Here's how the part is built. I have some questions about the finished solid (model axes, mm). A direction names the side the tool comes from. Coordinates: 2 decimals unless noted, no trailing zeros. Write each loop counter-clockwise with the first axis right and the second up, starting at its lowest first coordinate (ties: lowest second). Pieces come first, ordered by that corner, then holes. Notation, with made-up numbers: (66.25, 69.25) -> (94.25, 69.25) arc R20 cw to (94.25, 90.25) -> close; hole circle Ø9 at (-25.5, 34). An arc over 180 degrees is marked (long way). Use a Markdown table: item, result. Add a question column.
Item 1: Imagine slicing it at A-A, the plane x = 0. Write out the boundary of the cut face in (y, z).
Item 2: Will these pins go through, and if not, where does the flat tip stop? pin 1 Ø4 at (x, z) = (-36, -63) entering from +Y; pin 2 Ø2 at (x, z) = (-5, 24.3) entering from +Y; pin 3 Ø8 at (y, z) = (9, 56) entering from +X; pin 4 Ø6 at (x, z) = (-74.65, 0) entering from +Y.
Item 3: If I drill on line 1 along X through (y, z) = (3, 0); line 2 along X through (y, z) = (26, 34); line 3 along Z through (x, y) = (5, 25.5), over which ranges is the centre line in solid material (lowest first)? Write a range as from..to.
Item 4: Imagine slicing it at C-C, the plane z = 47.5. Write out the boundary of the cut face in (x, y).
Item 5: On a 3-axis mill with a long thin cutter (end or side, diameter ignored), from which of +Z, -Z, +X, -X, +Y, -Y can I reach the whole of each face in a straight line? I mean faces 1 (the flat face through (0, 20, 20.574)), 2 (the flat face through (-10.16, 5, -1)), 3 (the flat face through (43, 53.34, -29)). Say none if no direction works.
Item 6: Imagine slicing it at B-B, the plane z = 0. Write out the boundary of the cut face in (x, y).
Item 7: Imagine slicing it at D-D, the plane y = 35. Write out the boundary of the cut face in (x, z).
Item 8: If we mould it in two halves opening along Z, with no side actions, what happens to faces 4 (the flat face through (61.13, 6.858, 17.84)), 5 (the flat face through (0, 7.366, 0)), 6 (the cylindrical face through (81.318, 3.381, -10.677))? For each: pulls with the +Z half, pulls with the -Z half, needs draft (parallel to the pull), parting line crosses it, or undercut.
```python
from build123d import *

# Parameters (mm, degrees)
SKETCH2_R                       = 63.5
SKETCH2_R_2                     = 50.8
BOSS_EXTRUDE1_DEPTH             = 53.34
SKETCH4_R                       = 82.015423661
BOSS_EXTRUDE3_DEPTH             = 6.858
CUT_EXTRUDE2_DEPTH              = 125.954534773
CUT_EXTRUDE2_DEPTH_BACK         = 125.954534773
SKETCH6_R                       = 5.121456342
CUT_EXTRUDE3_DEPTH              = 125.954534773
CUT_EXTRUDE3_DEPTH_BACK         = 125.954534773
SKETCH9_W                       = 20.32
SKETCH9_H                       = 38.475908221
BOSS_EXTRUDE4_DEPTH             = 25.908
CUT_EXTRUDE5_DEPTH              = 121.526636859
CUT_EXTRUDE5_DEPTH_BACK         = 25.4
SKETCH11_W                      = 20.32
SKETCH11_H                      = 41.148
FILLET1_R                       = 1.27
M4X0_7_TAPPED_HOLE3_D           = 3.3
M4X0_7_TAPPED_HOLE3_DEPTH       = 9.906
M4X0_7_TAPPED_HOLE3_CSINK_D     = 4.05
M4X0_7_TAPPED_HOLE3_CSINK_ANGLE = 100
M4X0_7_TAPPED_HOLE3_TIP         = 0.991420021


with BuildPart() as part:
    # Sketch2 → Boss-Extrude1 (new body)
    with BuildSketch(Plane(origin=(0, 0, 0), x_dir=(1, 0, 0), z_dir=(0, 1, 0))):
        with Locations(Location((0, 0, 0), (0, 0, 270))):
            Circle(SKETCH2_R)
        with Locations(Location((0, 0, 0), (0, 0, 270))):
            Circle(SKETCH2_R_2, mode=Mode.SUBTRACT)
    extrude(amount=BOSS_EXTRUDE1_DEPTH)

    # Sketch4 → Boss-Extrude3 (add)
    with BuildSketch(Plane(origin=(0, 0, 0), x_dir=(1, 0, 0), z_dir=(0, 1, 0))):
        with Locations(Location((0, 0, 0), (0, 0, 270))):
            Circle(SKETCH4_R)
    extrude(amount=BOSS_EXTRUDE3_DEPTH)

    # Sketch6 → Cut-Extrude2 (cut, two sides: drawn at the far end of the back side and taken through both)
    with BuildSketch(Plane(origin=(0, 6.858, 0), x_dir=(1, 0, 0), z_dir=(0, 1, 0)).offset(-CUT_EXTRUDE2_DEPTH_BACK)):
        with Locations(Location((0, 74.395423661, 0), (0, 0, 270))):
            Circle(SKETCH6_R)
        with Locations(Location((-74.649423661, 0, 0), (0, 0, 270))):
            Circle(SKETCH6_R)
        with Locations(Location((74.395423661, 0, 0), (0, 0, 270))):
            Circle(SKETCH6_R)
        with Locations(Location((0, -74.395423661, 0), (0, 0, 270))):
            Circle(SKETCH6_R)
    extrude(amount=CUT_EXTRUDE2_DEPTH + CUT_EXTRUDE2_DEPTH_BACK, mode=Mode.SUBTRACT)

    # Sketch8 → Cut-Extrude3 (cut, two sides: drawn at the far end of the back side and taken through both)
    with BuildSketch(Plane(origin=(0, 6.858, 0), x_dir=(1, 0, 0), z_dir=(0, 1, 0)).offset(-CUT_EXTRUDE3_DEPTH_BACK)):
        with BuildLine():
            Line((-10.16, 49.773631573), (-10.16, -49.773631573))
            ThreePointArc((-10.16, -49.773631573), (-50.8, 0), (-10.16, 49.773631573))
        make_face()
        with BuildLine():
            Line((10.16, 49.773631573), (10.16, -49.773631573))
            ThreePointArc((10.16, -49.773631573), (50.8, 0), (10.16, 49.773631573))
        make_face()
    extrude(amount=CUT_EXTRUDE3_DEPTH + CUT_EXTRUDE3_DEPTH_BACK, mode=Mode.SUBTRACT)

    # Sketch9 → Boss-Extrude4 (add)
    with BuildSketch(Plane(origin=(0, 6.858, 0), x_dir=(1, 0, 0), z_dir=(0, 1, 0))):
        with Locations((0, 30.667954111)):
            Rectangle(SKETCH9_W, SKETCH9_H)
        with BuildLine():
            Line((-10.16, 49.773631573), (-10.16, -49.773631573))
            ThreePointArc((-10.16, -49.773631573), (0, -50.8), (10.16, -49.773631573))
            Line((10.16, -49.773631573), (10.16, 49.773631573))
            ThreePointArc((10.16, 49.773631573), (0, 50.8), (-10.16, 49.773631573))
        make_face()
    extrude(amount=BOSS_EXTRUDE4_DEPTH)

    # Sketch11 → Cut-Extrude5 (cut, two sides: drawn at the far end of the back side and taken through both)
    with BuildSketch(Plane(origin=(0, 32.766, 0), x_dir=(1, 0, 0), z_dir=(0, 1, 0)).offset(-CUT_EXTRUDE5_DEPTH_BACK)):
        Rectangle(SKETCH11_W, SKETCH11_H)
    extrude(amount=CUT_EXTRUDE5_DEPTH + CUT_EXTRUDE5_DEPTH_BACK, mode=Mode.SUBTRACT)

    # Fillet1
    fillet1_edges = [part.edges().sort_by_distance(p)[0] for p in [
        (0, 32.766, 20.574),
        (0, 7.366, 20.574),
        (0, 7.366, -20.574),
        (0, 32.766, -20.574),
    ]]
    fillet(fillet1_edges, radius=FILLET1_R)

    # M4x0.7 Tapped Hole3
    with Locations(Plane(origin=(0, 32.766, 0), x_dir=(1, 0, 0), z_dir=(0, 1, 0))):
        with Locations((5, -24.3), (-5, -24.3), (5, 24.3), (-5, 24.3)):
            CounterSinkHole(M4X0_7_TAPPED_HOLE3_D / 2, M4X0_7_TAPPED_HOLE3_CSINK_D / 2, depth=M4X0_7_TAPPED_HOLE3_DEPTH, counter_sink_angle=M4X0_7_TAPPED_HOLE3_CSINK_ANGLE)
            with Locations((0, 0, -(M4X0_7_TAPPED_HOLE3_DEPTH + M4X0_7_TAPPED_HOLE3_TIP / 2))):  # 118° drill point
                Cone(0, M4X0_7_TAPPED_HOLE3_D / 2, M4X0_7_TAPPED_HOLE3_TIP, mode=Mode.SUBTRACT)


solid = part.part
```
Ans:
| question | item | result |
|---|---|---|
| 1 | outline | (0, -82.02) -> (6.86, -82.02) -> (6.86, -79.52) -> (0, -79.52) -> close; (0, -69.27) -> (6.86, -69.27) -> (6.86, -63.5) -> (53.34, -63.5) -> (53.34, -50.8) -> (32.77, -50.8) -> (32.77, -21.84) arc R1.27 ccw to (31.5, -20.57) -> (8.64, -20.57) arc R1.27 cw to (7.37, -19.3) -> (7.37, 19.3) arc R1.27 cw to (8.64, 20.57) -> (31.5, 20.57) arc R1.27 ccw to (32.77, 21.84) -> (32.77, 50.8) -> (53.34, 50.8) -> (53.34, 63.5) -> (6.86, 63.5) -> (6.86, 69.27) -> (0, 69.27) -> close; (0, 79.52) -> (6.86, 79.52) -> (6.86, 82.02) -> (0, 82.02) -> close |
| 2 | pin 1 | stops at y = 6.86 |
| 2 | pin 2 | stops at y = 22.47 |
| 2 | pin 3 | stops at x = 62.91 |
| 2 | pin 4 | passes through |
| 3 | line 1 | x = -82.02..-79.77, -69.53..-50.8, -10.16..10.16, 50.8..69.27, 79.52..82.02 |
| 3 | line 2 | x = -53.63..-37.74, -10.16..10.16, 37.74..53.63 |
| 3 | line 3 | z = -63.3..-25.95, -22.65..-20.57, 20.57..22.65, 25.95..63.3 |
| 4 | outline | (-66.86, 0) -> (-18.01, 0) -> (-18.01, 53.34) -> (-42.14, 53.34) -> (-42.14, 6.86) -> (-66.86, 6.86) -> close; (-10.16, 0) -> (10.16, 0) -> (10.16, 32.77) -> (-10.16, 32.77) -> close; (18.01, 0) -> (66.86, 0) -> (66.86, 6.86) -> (42.14, 6.86) -> (42.14, 53.34) -> (18.01, 53.34) -> close |
| 5 | face 1 | +Y |
| 5 | face 2 | +Y, -Y |
| 5 | face 3 | +Z, -Z, +X, -X, +Y |
| 6 | outline | (-82.02, 0) -> (-79.77, 0) -> (-79.77, 6.86) -> (-82.02, 6.86) -> close; (-69.53, 0) -> (-50.8, 0) -> (-50.8, 53.34) -> (-63.5, 53.34) -> (-63.5, 6.86) -> (-69.53, 6.86) -> close; (-10.16, 0) -> (10.16, 0) -> (10.16, 7.37) -> (-10.16, 7.37) -> close; (50.8, 0) -> (69.27, 0) -> (69.27, 6.86) -> (63.5, 6.86) -> (63.5, 53.34) -> (50.8, 53.34) -> close; (79.52, 0) -> (82.02, 0) -> (82.02, 6.86) -> (79.52, 6.86) -> close |
| 7 | outline | circle Ø127 at (0, 0); hole circle Ø101.6 at (0, 0) |
| 8 | face 4 | needs draft |
| 8 | face 5 | undercut |
| 8 | face 6 | parting line crosses it |
